Input: part model. Units: mm. Frame: model coordinates. Face numbers are marked on the shaded views. Give positions to 0.01 mm unless a question says otherwise; leave off trailing zeros. Loops run counter-clockwise (first coordinate to the right, second up) from the corner with the lowest first, then second, coordinate; pieces in that order, holes last. Notation, with made-up numbers: (49, -31.75) -> (85, -31.75) arc R31 ccw to (85, 2.25) -> close; hole circle Ø8 at (13.5, 50.5). An arc over 180 degrees is marked (long way). Answer as a JSON object with one key per item and string values.
```python
from build123d import *

# Parameters (mm, degrees)
CYLINDER003_R     = 4
CYLINDER003_DEPTH = 10
PRISM_DEPTH       = 2
CYLINDER002_R     = 5
CYLINDER002_DEPTH = 1.5
CHAMFER002_SIZE   = 1


with BuildPart() as cylinder003:
    # Cylinder003 → Cylinder003 (new body)
    with BuildSketch(Plane.XY.offset(-1)):
        Circle(CYLINDER003_R)
    extrude(amount=CYLINDER003_DEPTH)


with BuildPart() as prism:
    # Prism → Prism (new body)
    with BuildSketch(Plane.XY):
        Polygon((7, 0), (3.5, 6.062178), (-3.5, 6.062178), (-7, 0), (-3.5, -6.062178), (3.5, -6.062178), align=None)
    extrude(amount=PRISM_DEPTH)


with BuildPart() as cut003:
    # Cylinder002 → Cylinder002 (new body)
    with BuildSketch(Plane.XY.offset(1)):
        Circle(CYLINDER002_R)
    extrude(amount=CYLINDER002_DEPTH)

    # Chamfer002
    chamfer002_edges = [cut003.edges().sort_by_distance(p)[0] for p in [
        (-5, 0, 2.5),
    ]]
    chamfer(chamfer002_edges, length=CHAMFER002_SIZE)

    # Fusion006: union Prism
    add(prism.part)

    # Cut003: cut Cylinder003
    add(cylinder003.part, mode=Mode.SUBTRACT)


solid = cut003.part
```
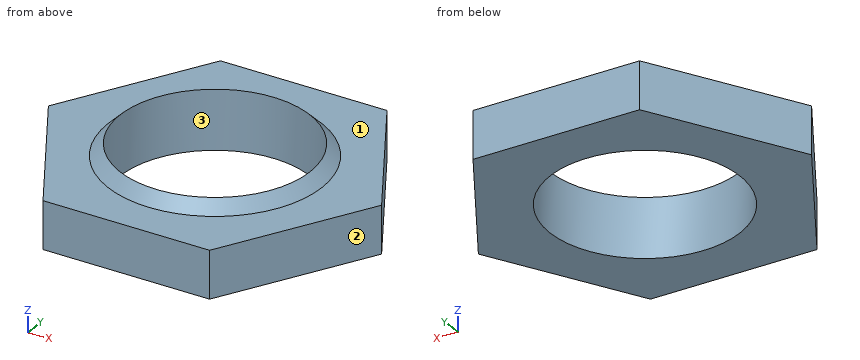
Q1. Section A-A, the plane z = 0.9. Return the cut outline in (x, y), then the cut area to 3 significant figures.
Evaluation:
{"outline": "(-7, 0) -> (-3.5, -6.06) -> (3.5, -6.06) -> (7, 0) -> (3.5, 6.06) -> (-3.5, 6.06) -> close; hole circle Ø8 at (0, 0)", "area": "77.0 mm2"}
Q2. Ray query, line 1 along Y through (x, z) = (0, 1.35); line 2 along X through (y, z) = (1.25, 1.55); line 3 along X through (y, z) = (0.75, 1.85). Return the intervals inside material, ascending.
Evaluation:
{"line 1": "y = -6.06 to -4, 4 to 6.06", "line 2": "x = -6.28 to -3.8, 3.8 to 6.28", "line 3": "x = -6.57 to -3.93, 3.93 to 6.57"}
Q3. Section D-D, the plane y = 5. Return the cut outline in (x, z), then the cut area to 3 significant figures.
Evaluation:
{"outline": "(-4.11, 0) -> (4.11, 0) -> (4.11, 2) -> (-4.11, 2) -> close", "area": "16.5 mm2"}
Q4. Pin query (flat end, axial travel): pin 1 (1 mm diameter, centred on y = 2.5, z = 0.5, fed in from -X); pin 2 (6 mm diameter, centred on x = 3, y = -0.5, fed in from -Z). Return the tip coordinate at first contact, or that it passes through.
Evaluation:
{"pin 1": "stops at x = -5.85", "pin 2": "stops at z = 0"}
Q5. Draft query along Y for the marked faces 1, 2 and 3. Return one class per face: +Y half, -Y half, draft (parallel to the pull), parting line (faces both ways), or undercut.
Evaluation:
{"face 1": "draft", "face 2": "-Y half", "face 3": "undercut"}
Q6. Section B-B, the plane x = 0. Return the cut outline in (y, z).
Evaluation:
{"outline": "(-6.06, 0) -> (-4, 0) -> (-4, 2.5) -> (-4.5, 2) -> (-6.06, 2) -> close; (4, 0) -> (6.06, 0) -> (6.06, 2) -> (4.5, 2) -> (4, 2.5) -> close"}
